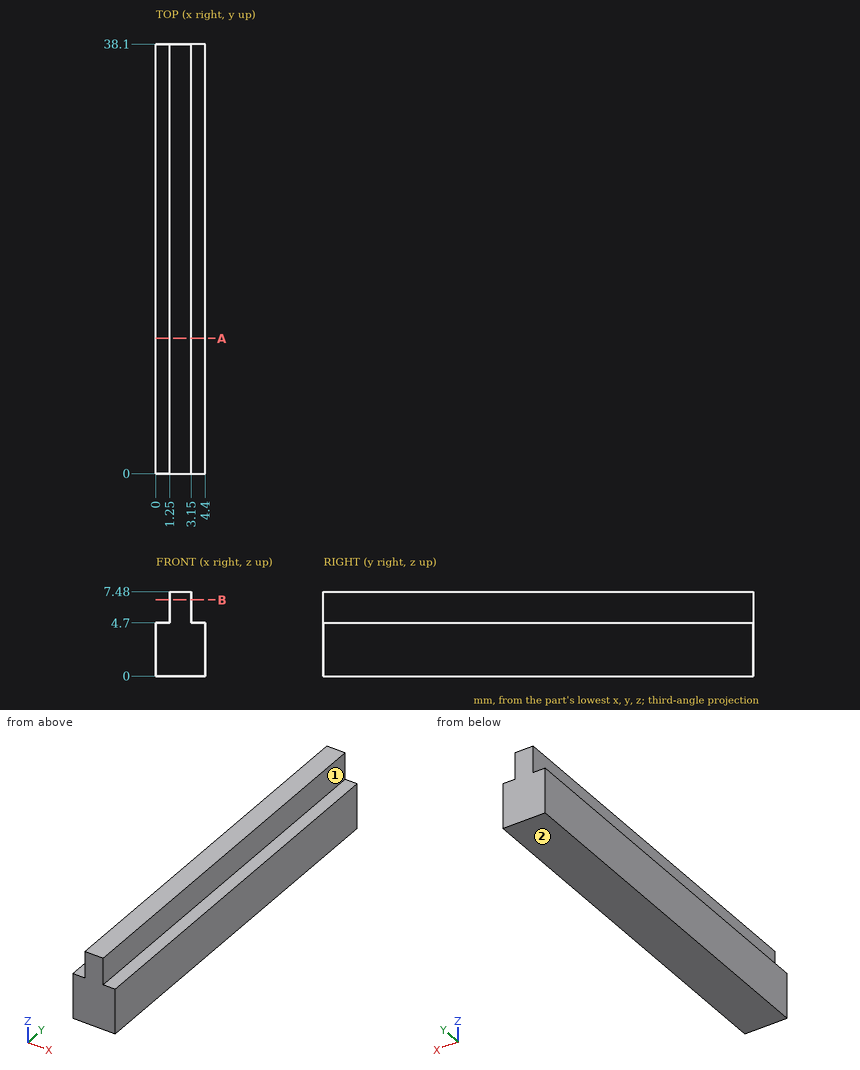
Check sheet for the drawn part. Datum: minimum x, y, z corner. Units: mm. A direction names the side the tool comes from. Give positions to 0.01 mm unless a question says otherwise; leave off trailing zeros. Order: outer loops, then holes, each group sorted by start corner. A loop starts at its lowest first (then second) coordinate and runs counter-clockwise, first axis right, second up.
1. Sectioned sample at A-A (y = 12). Record the boundary of the cut face in (x, z), then the cut area to 3 significant figures.
Completed:
outline: (0, 0) - (4.4, 0) - (4.4, 4.7) - (3.15, 4.7) - (3.15, 7.48) - (1.25, 7.48) - (1.25, 4.7) - (0, 4.7) - close
area: 26.0 mm2
2. Sectioned sample at B-B (z = 6.75). Record the boundary of the cut face in (x, y).
Completed:
outline: (1.25, 0) - (3.15, 0) - (3.15, 38.1) - (1.25, 38.1) - close
3. Depth check by flat-ended pin: pin 1 (1.4 mm diameter, centred on y = 23, z = 6, fed in from -X); pin 2 (1.4 mm diameter, centred on x = 4, y = 13.5, fed in from +Z). Enter the tip coordinate at first touch or a pass-through.
Completed:
pin 1: stops at x = 1.25
pin 2: stops at z = 4.7
4. Access from +Z, -Z, +X, -X, +Y, -Y to the whole of each face (thin tool, end or side, straight path). Record for the marked faces 1 and 2.
Completed:
face 1: +Z, +X, +Y, -Y
face 2: -Z, +X, -X, +Y, -Y
5. Scan lines: line 1 (Z direction, x = 4.05, y = 4); line 2 (X direction, y = 8.5, z = 6.75). Record each from-to range of solid material in increasing order.
Completed:
line 1: z = 0 to 4.7
line 2: x = 1.25 to 3.15
